Solid Edge part; units mm, degrees
sketch "Sketch1" plane through (0, 0, 0) normal (1, 0, 0) x (0, 1, 0)
  circle A0 centre (0, 0) radius 125
  circle A1 centre (0, 0) radius 26
extrude "Protrusion1" add sketch "Sketch1" along normal mid plane 80
sketch "Sketch2" plane through (40, 0, 0) normal (1, 0, 0) x (0, 1, 0)
  circle A0 centre (0, 0) radius 50
extrude "Extrusionsausschnitt_1" cut sketch "Sketch2" against normal blind 38
chamfer "Fase_1" distance 20 angle 45 1 edges at (40, -50, 0)
fillet "Verrundung_1" radius 30 1 edges at (40, -125, 0)
mirror "Mirror1" about plane through (0, 0, 0) normal (1, 0, 0) of "Extrusionsausschnitt_1", "Fase_1", "Verrundung_1"
sketch "Sketch3" plane through (2, 0, 0) normal (1, 0, 0) x (0, 1, 0)
  circle A0 centre (0, 35) radius 4.25
  circle A1 centre (35, 0) radius 4.25
  circle A2 centre (0, -35) radius 4.25
  circle A3 centre (-35, 0) radius 4.25
extrude "Extrusionsausschnitt_2" cut sketch "Sketch3" against normal blind 295
sketch "Sketch4" plane through (2, 0, 0) normal (1, 0, 0) x (0, 1, 0)
  circle A0 centre (24.7487, 24.7487) radius 7.5
  circle A1 centre (-24.7487, 24.7487) radius 7.5
  circle A2 centre (24.7487, -24.7487) radius 7.5
  circle A3 centre (-24.7487, -24.7487) radius 7.5
extrude "Extrusionsausprägung_2" add sketch "Sketch4" along normal blind 10
mirror "Mirror2" about plane through (0, 0, 0) normal (1, 0, 0) of "Extrusionsausprägung_2"
Build history of the part. All positions in model axes, mm. A direction names the side the tool comes from. Round coordinates to 2 decimals unless told otherwise and drop trailing zeros. Loops run counter-clockwise (first coordinate to the right, second up) from the corner with the lowest first, then second, coordinate; pieces in that order, holes last. Notation, with made-up numbers: (18, -25) -> (76, -25) arc R30 cw to (76, -3) -> close; hole circle Ø10 at (71.25, 49.5). An arc over 180 degrees is marked (long way). One line per item, written item: value. Start each with the question number.
Q1. Two-plate mould, pull along Y, no slides. Class faces 4 (the face through (-40, 70, -7)), 5 (the face through (-21.25, -11.11, 50.03)): released by +Y, released by -Y, zero draft, split by the parting line, or undercut.
Q2. Cut at C-C on x = -32. List the corners of the cut face in (y, z), plus the area to 3 significant figures.
Q3. Cut at A-A on y = 0. Count the separate pieces of the cut face and the enclosed holes in it, plus the area to 3 significant figures.
Q4. Drop flat-ended pins along their axis: pin 1 Ø4.5 at (y, z) = (22, 24.5) entering from +X; pin 2 Ø4.5 at (y, z) = (22, -23.5) entering from -X; pin 3 Ø13.5 at (y, z) = (35, 0) entering from -X. Give the stop position or say it passes through.
Q5. Probe line 1 along Z through (x, y) = (-4, 28); line 2 along Z through (x, y) = (11.5, 0); line 3 along Z through (x, y) = (11.5, 29). List the from-to ranges inside material, lowest first.
Q6. Cut at B-B on x = -7. List the corners of the cut face in (y, z).
Q7. 3-axis set-ups, long thin cutter, end or side, ignore diameter. For faces 1 (the face through (6.93, -17.595, -27.001)), 2 (the face through (-12, 25, -25)), 3 (the face through (0.028, 30.754, 0.187)): which of +Z, -Z, +X, -X, +Y, -Y reach the whole face in a straight line?
Computed:
1. face 4: zero draft
1. face 5: undercut
2. outline: circle Ø230.79 at (0, 0); hole circle Ø124 at (0, 0)
2. area: 29,800 mm²
3. separate pieces: 4
3. enclosed holes: 0
3. area: 10,600 mm²
4. pin 1: x = 12
4. pin 2: x = -12
4. pin 3: x = -2
5. line 1: -121.82 to -41.42, -31.51 to -17.99, 17.99 to 31.51, 41.42 to 121.82
5. line 2: -124.96 to -50, 50 to 124.96
5. line 3: -121.55 to -40.73, -30.93 to -18.57, 18.57 to 30.93, 40.73 to 121.55
6. outline: circle Ø250 at (0, 0); circle Ø15 at (-24.75, -24.75); circle Ø15 at (-24.75, 24.75); circle Ø15 at (24.75, -24.75); circle Ø15 at (24.75, 24.75); hole circle Ø100 at (0, 0)
7. face 1: +X
7. face 2: -X
7. face 3: +X, -X
